Design review of the part built by this model. Coordinates are the model's own, in mm. A direction names the side the tool comes from. Give positions to 0.01 mm unless a question says otherwise; leave off trailing zeros. Loops run counter-clockwise (first coordinate to the right, second up) from the corner with the lowest first, then second, coordinate; pieces in that order, holes last. Notation, with made-up numbers: M 52,51.25 L 86,51.25 A26 cw 86,76.25 Z; hole C 42,-39.75 d4. An arc over 180 degrees is marked long. Answer as CSV lines item,"result".
```python
from build123d import *

# Parameters (mm, degrees)
F1_DEPTH = 15
F3_DEPTH = 6


with BuildPart() as f1:
    # F0 (on Top) → F1 (new body)
    with BuildSketch(Plane.XY):
        Polygon((-85.244147, 33.927911), (-93.244147, 33.927911), (-93.244147, 19.927911), (-93.244147, 13.927911), (-83.244147, 13.927911), (-83.244147, 19.927911), (-73.244147, 19.927911), (-73.244147, 29.927911), (-83.244147, 29.927911), (-83.244147, 33.927911), align=None)
    extrude(amount=F1_DEPTH)

    # F2 (on face) → F3 (join)
    with BuildSketch(Plane.XY.offset(15)):
        Polygon((-85.244147, 19.927911), (-85.244147, 13.927911), (-83.244147, 13.927911), (-83.244147, 19.927911), (-73.244147, 19.927911), (-73.244147, 21.978136), (-85.244147, 21.978136), align=None)
        Polygon((-91.244147, 33.927911), (-93.244147, 33.927911), (-93.244147, 31.927911), (-93.244147, 13.927911), (-91.244147, 13.927911), (-91.244147, 31.927911), (-85.244147, 31.927911), (-85.244147, 29.927911), (-85.244147, 27.927911), (-73.244147, 27.927911), (-73.244147, 29.927911), (-83.244147, 29.927911), (-83.244147, 31.927911), (-83.244147, 33.927911), (-85.244147, 33.927911), align=None)
    extrude(amount=F3_DEPTH)


solid = f1.part
```
1. We need section A-A, the plane x = -84.25. Write out the cut boundary in (y, z).
Answer block:
outline,"M 13.93,0 L 33.93,0 L 33.93,21 L 27.93,21 L 27.93,15 L 21.98,15 L 21.98,21 L 13.93,21 Z"
2. We need section C-C, the plane y = 22.75. Write out the cut boundary in (x, z).
Answer block:
outline,"M -93.24,0 L -73.24,0 L -73.24,15 L -91.24,15 L -91.24,21 L -93.24,21 Z"
3. To check wall thickness, follow L1, parallel to Y at x = -75.5, z = 16; L2, parallel to X at y = 19.25, z = 16.75; L3, parallel to Z at x = -90.75, y = 27.25. State the ranges of each line that lie inside material, in increasing order. Write a range as [from, to].
Answer block:
L1,"[19.93, 21.98], [27.93, 29.93]"
L2,"[-93.24, -91.24], [-85.24, -83.24]"
L3,"[0, 15]"
4. We need section B-B, the plane y = 31.5. Write out the cut boundary in (x, z), plus the area to 3 significant figures.
Answer block:
outline,"M -93.24,0 L -83.24,0 L -83.24,21 L -85.24,21 L -85.24,15 L -91.24,15 L -91.24,21 L -93.24,21 Z"
area,"174 mm²"
5. For faces 1 (the flat face through (-83.244, 17, 10)), 2 (the flat face through (-88, 31.928, 18)), 3 (the flat face through (-78, 29.928, 10)), 4 (the flat face through (-79, 27.928, 18)), list the 3-axis set-ups (+Z, -Z, +X, -X, +Y, -Y) from which the entire face can be reached by the end or side of a thin tool; tool diameter is ignored.
Answer block:
face 1,"+Z, -Z, +X, -Y"
face 2,"+Z, -Y"
face 3,"+Z, -Z, +X, +Y"
face 4,"+Z, +X"
6. The part is to be moulded in two halves that separate along X. For faces 5 (the flat face through (-84, 23, 15)), 6 (the flat face through (-83.244, 32, 10)), 7 (the flat face through (-91.244, 23, 18)), 8 (the flat face through (-78, 19.928, 10)), say which applies: pulls with the +X half, pulls with the -X half, needs draft (parallel to the pull), parting line crosses it, or undercut.
Answer block:
face 5,"undercut"
face 6,"pulls with the +X half"
face 7,"undercut"
face 8,"needs draft"
7. For P1, Ø1.2, axis at y = 31, z = 6, coming from the +X side; P2, Ø5, axis at x = -77, z = 18, coming from the -Y side; P3, Ø3, axis at x = -87.5, z = 18.5, coming from the -Y side, all flat-tipped, find the tip position at first contact; note any pin that passes through.
Answer block:
P1,"x = -83.24"
P2,"y = 19.93"
P3,"y = 31.93"
